Geometry: final body of the model. Coordinates: model frame, mm. A direction names the side the tool comes from. Give positions to 0.01 mm unless a question says otherwise; leave off trailing zeros. Order: outer loops, then holes, each group sorted by start corner. A loop starts at its lowest first (then second) coordinate and runs counter-clockwise, first axis right, second up. Notation, with made-up numbers: (74, 62.25) -> (96, 62.25) arc R10 ccw to (96, 69.25) -> close; hole circle Ø4 at (70.25, -33.75). An arc over 180 degrees is marked (long way). One line per question, with ' | ' between items. Start each with the question number.
(1) Section A-A (y = 3.5). Return loops of the section in (x, z), then the cut area to 3 significant figures.
(2) Mould query, pull axis X, two halves, no side actions, for faces 5 (the face through (-189, -1, -97.5)), 6 (the face through (-130, -1, -34)), 7 (the face through (-219, -2, -4.505)). Classes: +X half, -X half, draft (parallel to the pull), parting line (faces both ways), or undercut.
(3) Section B-B (x = -161). Return loops of the section in (y, z), then the cut area to 4 significant figures.
(4) Set-up query: faces 1 (the face through (-185.347, 3.451, -89.068)), 2 (the face through (-232, -2, -4.505)), 3 (the face through (-189, 5, -3)), 4 (the face through (-191, 7, 24)). Return all of +Z, -Z, +X, -X, +Y, -Y with unobstructed straight access to the full face (end or side cutting, diameter ignored); none if empty.
(5) Ray query, L1, parallel to Z at x = -219.5, y = -0.5; L2, parallel to X at y = 2.75, z = -48.5; L3, parallel to Z at x = -214, y = 5.5. Return the intervals inside material, ascending.
(6) Section D-D (x = -146.5). Return loops of the section in (y, z), then the cut area to 3 significant figures.
(7) First-contact query: pin 1 Ø12 at (x, z) = (-148.5, -50.5) entering from +Y; pin 2 Ø3.5 at (x, z) = (-173.5, -7) entering from +Y. Flat tips, straight axial feed; report the tip coordinate or a pass-through.
(8) Section C-C (z = -48.5). Return loops of the section in (x, y), then the cut area to 3 significant figures.
```python
from build123d import *

# Parameters (mm, degrees)
SKETCH1_W           = 120
SKETCH1_H           = 55
BOSS_EXTRUDE1_DEPTH = 5
SKETCH2_W           = 120
SKETCH2_H           = 7.5
BOSS_EXTRUDE2_DEPTH = 20
SKETCH3_W           = 120
SKETCH3_H           = 2.5
BOSS_EXTRUDE4_DEPTH = 20
BOSS_EXTRUDE5_DEPTH = 190
SKETCH9_W           = 310
SKETCH9_H           = 25
BOSS_EXTRUDE6_DEPTH = 70
SKETCH14_R          = 5.5
CUT_EXTRUDE5_DEPTH  = 153
SKETCH15_W          = 125
SKETCH15_H          = 25
CUT_EXTRUDE6_DEPTH  = 190
SKETCH16_W          = 120
SKETCH16_H          = 125
BOSS_EXTRUDE8_DEPTH = 10
SKETCH17_W          = 120
SKETCH17_H          = 125
CUT_EXTRUDE7_DEPTH  = 18
CUT_EXTRUDE8_START  = -31
SKETCH18_R          = 5.5
CUT_EXTRUDE8_DEPTH  = 31
SKETCH19_W          = 15.5
SKETCH19_H          = 5.5
CUT_EXTRUDE9_DEPTH  = 31


with BuildPart() as part:
    # Sketch1 → Boss-Extrude1 (new body)
    with BuildSketch(Plane(origin=(0, 0, 0), x_dir=(1, 0, 0), z_dir=(0, 1, 0))):
        Rectangle(SKETCH1_W, SKETCH1_H)
    extrude(amount=BOSS_EXTRUDE1_DEPTH)

    # Sketch2 → Boss-Extrude2 (add)
    with BuildSketch(Plane(origin=(0, 5, 0), x_dir=(1, 0, 0), z_dir=(0, 1, 0))):
        with Locations((0, -23.75)):
            Rectangle(SKETCH2_W, SKETCH2_H)
    extrude(amount=BOSS_EXTRUDE2_DEPTH)

    # Sketch3 → Boss-Extrude4 (add)
    with BuildSketch(Plane(origin=(0, 5, 0), x_dir=(1, 0, 0), z_dir=(0, 1, 0))):
        with Locations((0, 26.25)):
            Rectangle(SKETCH3_W, SKETCH3_H)
    extrude(amount=BOSS_EXTRUDE4_DEPTH)

    # Sketch8 → Boss-Extrude5 (add)
    with BuildSketch(Plane.ZY.offset(60)):
        Polygon((-27.5, 0), (-27.5, 25), (-25, 25), (-25, 5), (20, 5), (20, 25), (27.5, 25), (27.5, 0), align=None)
    extrude(amount=BOSS_EXTRUDE5_DEPTH)

    # Sketch9 → Boss-Extrude6 (add)
    with BuildSketch(Plane(origin=(0, 0, -27.5), x_dir=(-1, 0, 0), z_dir=(0, 0, -1))):
        with Locations((95, 12.5)):
            Rectangle(SKETCH9_W, SKETCH9_H)
    extrude(amount=BOSS_EXTRUDE6_DEPTH)

    # Sketch14 → Cut-Extrude5 (cut)
    with BuildSketch(Plane(origin=(0, 0, 0), x_dir=(-1, 0, 0), z_dir=(0, -1, 0))):
        with Locations(Location((225.445279058, 7.255161462, 0), (0, 0, 90))):
            Circle(SKETCH14_R)
        with Locations(Location((175.445279058, 7.255161462, 0), (0, 0, 90))):
            Circle(SKETCH14_R)
        with Locations(Location((225.445279058, 57.255161462, 0), (0, 0, 90))):
            Circle(SKETCH14_R)
        with Locations(Location((148.0182107, 48.5, 0), (0, 0, 90))):
            Circle(SKETCH14_R)
        with Locations(Location((183.240850763, 83.987541856, 0), (0, 0, 90))):
            Circle(SKETCH14_R)
    extrude(amount=-CUT_EXTRUDE5_DEPTH, mode=Mode.SUBTRACT)

    # Sketch15 → Cut-Extrude6 (cut)
    with BuildSketch(Plane(origin=(60, 0, 0), x_dir=(0, 0, -1), z_dir=(1, 0, 0))):
        with Locations((35, 12.5)):
            Rectangle(SKETCH15_W, SKETCH15_H)
    extrude(amount=-CUT_EXTRUDE6_DEPTH, mode=Mode.SUBTRACT)

    # Sketch16 → Boss-Extrude8 (add)
    with BuildSketch(Plane(origin=(0, 0, 0), x_dir=(-1, 0, 0), z_dir=(0, -1, 0))):
        with Locations((190, 35)):
            Rectangle(SKETCH16_W, SKETCH16_H)
    extrude(amount=BOSS_EXTRUDE8_DEPTH)

    # Sketch17 → Cut-Extrude7 (cut)
    with BuildSketch(Plane(origin=(0, 25, 0), x_dir=(1, 0, 0), z_dir=(0, 1, 0))):
        with Locations((-190, 35)):
            Rectangle(SKETCH17_W, SKETCH17_H)
    extrude(amount=-CUT_EXTRUDE7_DEPTH, mode=Mode.SUBTRACT)

    # Sketch18 → Cut-Extrude8 (cut)
    with BuildSketch(Plane(origin=(0, 5, 0), x_dir=(1, 0, 0), z_dir=(0, 1, 0)).offset(CUT_EXTRUDE8_START)):
        with Locations(Location((-225.445279058, 7.255161462, 0), (0, 0, 90))):
            Circle(SKETCH18_R)
    extrude(amount=CUT_EXTRUDE8_DEPTH, mode=Mode.SUBTRACT)

    # Sketch19 → Cut-Extrude9 (cut)
    with BuildSketch(Plane(origin=(0, 5, 0), x_dir=(1, 0, 0), z_dir=(0, 1, 0))):
        with Locations((-225.445279058, 7.255161462)):
            Rectangle(SKETCH19_W, SKETCH19_H)
    extrude(amount=-CUT_EXTRUDE9_DEPTH, mode=Mode.SUBTRACT)


solid = part.part
```
Response:
1) outline: (-250, -97.5) -> (-130, -97.5) -> (-130, 27.5) -> (-250, 27.5) -> close; hole (-233.2, -10.01) -> (-230.21, -10.01) arc R5.5 ccw to (-220.68, -10.01) -> (-217.7, -10.01) -> (-217.7, -4.51) -> (-220.68, -4.51) arc R5.5 ccw to (-230.21, -4.51) -> (-233.2, -4.51) -> close; hole circle Ø11 at (-225.45, -57.26); hole circle Ø11 at (-183.24, -83.99); hole circle Ø11 at (-175.45, -7.26); hole circle Ø11 at (-148.02, -48.5) | area: 14,500 mm^2
2) face 5: draft | face 6: +X half | face 7: undercut
3) outline: (-10, -97.5) -> (7, -97.5) -> (7, -25) -> (5, -25) -> (5, 20) -> (7, 20) -> (7, 27.5) -> (-10, 27.5) -> close | area: 2,035 mm^2
4) face 1: +Y | face 2: +Y, -Y | face 3: +X, -X, +Y | face 4: +Z, -Z, +X, -X, +Y
5) L1: z = -97.5 to -10.01, -4.51 to 27.5 | L2: x = -250 to -153.52, -142.52 to -130 | L3: z = -97.5 to -25, 20 to 27.5
6) outline: (-10, -97.5) -> (7, -97.5) -> (7, -53.79) -> (0, -53.79) -> (0, -43.21) -> (7, -43.21) -> (7, -25) -> (5, -25) -> (5, 20) -> (7, 20) -> (7, 27.5) -> (-10, 27.5) -> close | area: 1,960 mm^2
7) pin 1: stops at y = 7 | pin 2: stops at y = 0
8) outline: (-250, -10) -> (-130, -10) -> (-130, 7) -> (-142.52, 7) -> (-142.52, 0) -> (-153.52, 0) -> (-153.52, 7) -> (-250, 7) -> close | area: 1,960 mm^2
